Answer from the drawing. Dimensions are ordinates in mm from the lowest x, y and z of the part. Round coordinates to 2 decimals unless told otherwise and drop trailing zeros. Loops run counter-clockwise (first coordinate to the right, second up) from the corner with the lowest first, then second, coordinate; pieces in that order, holes last. Notation, with made-up numbers: M 25,44.25 L 33,44.25 A21 ccw 33,68.25 Z; hole C 68,4 d6. An arc over 180 degrees is marked long. Answer as a JSON object with one key per item and string values.
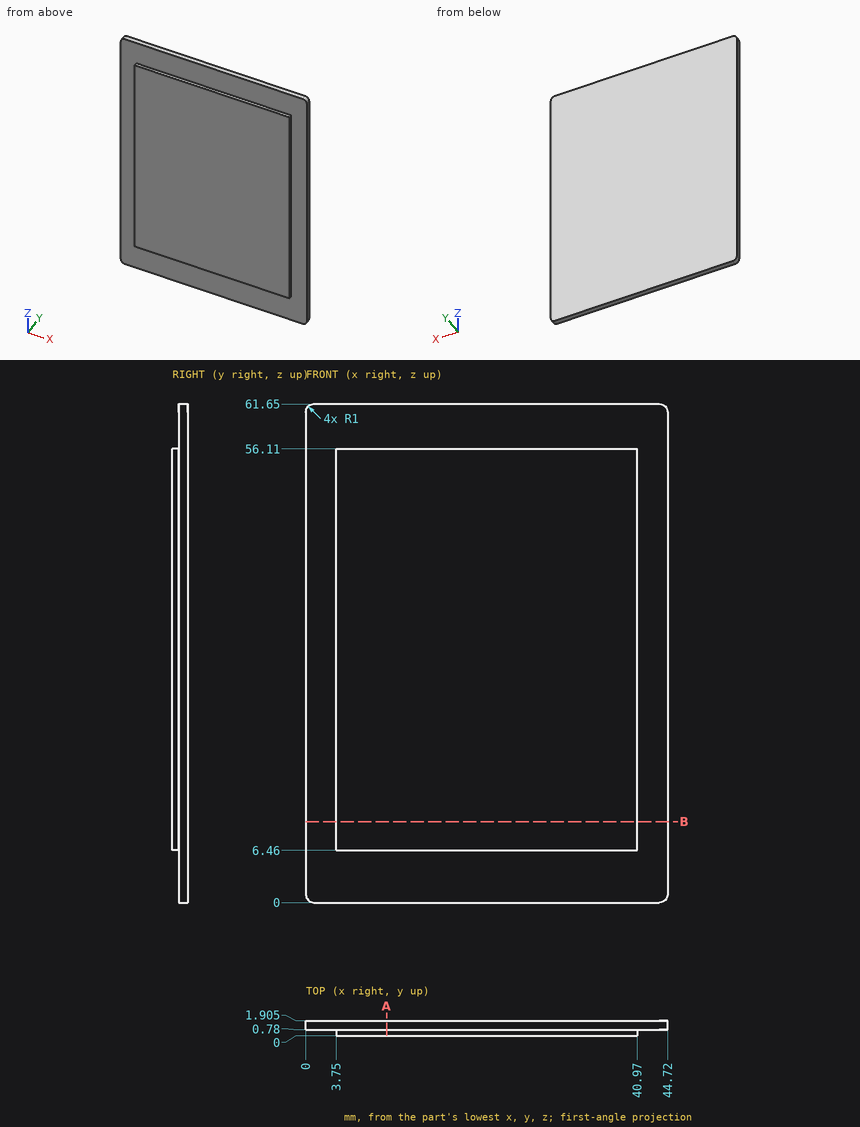
Item 1: Straight lines are drawn through the part: line 1 (Y direction, x = 24, z = 56.5) (3 decimals); line 2 (X direction, y = 0.2, z = 10); line 3 (Z direction, x = 15, y = 0.6). For each, find the intervals that lie inside material, in ascending order.
Values follow:
{"line 1": "0.78 to 1.905", "line 2": "3.75 to 40.97", "line 3": "6.46 to 56.11"}
Item 2: The part is cut by section B-B (z = 10). Give the vertices of the cut face in (x, y) (3 decimals), then the cut area to 3 significant figures.
Values follow:
{"outline": "M 0,0.78 L 3.75,0.78 L 3.75,0 L 40.97,0 L 40.97,0.78 L 44.72,0.78 L 44.72,1.905 L 0,1.905 Z", "area": "79.3 mm^2"}
Item 3: The part is cut by section A-A (x = 10). Give the vertices of the cut face in (y, z) (3 decimals), then the cut area to 3 significant figures.
Values follow:
{"outline": "M 0,6.46 L 0.78,6.46 L 0.78,0 L 1.905,0 L 1.905,61.65 L 0.78,61.65 L 0.78,56.11 L 0,56.11 Z", "area": "108 mm^2"}
